```python
from build123d import *

# Parameters (mm, degrees)
F0_R     = 14
F0_R_2   = 11
F1_DEPTH = 25
F0_R_3   = 33
F2_DEPTH = 5
F3_R     = 3
F4_DEPTH = 25
F6_R     = 1
F7_DEPTH = 2


with BuildPart() as f1:
    # F0 (on Top) → F1 (new body)
    with BuildSketch(Plane.XY):
        Circle(F0_R)
        Circle(F0_R_2, mode=Mode.SUBTRACT)
    extrude(amount=F1_DEPTH)

    # F0 (on Top) → F2 (join)
    with BuildSketch(Plane.XY):
        Circle(F0_R_3)
        Circle(F0_R, mode=Mode.SUBTRACT)
    extrude(amount=F2_DEPTH)

    # F3 (on Front) → F4 (cut)
    with BuildSketch(Plane.XZ):
        with Locations((0, 25)):
            Circle(F3_R)
    extrude(amount=-F4_DEPTH, mode=Mode.SUBTRACT)

    # F6 (on offset) → F7 (join)
    with BuildSketch(Plane.XY.offset(25)):
        with Locations((-8.8388347648, 8.8388347648)):
            Circle(F6_R)
        with Locations((8.8388347648, 8.8388347648)):
            Circle(F6_R)
        with Locations((12.5, 0)):
            Circle(F6_R)
        with Locations((8.8388347648, -8.8388347648)):
            Circle(F6_R)
        with Locations((0, -12.5)):
            Circle(F6_R)
        with Locations((-8.8388347648, -8.8388347648)):
            Circle(F6_R)
        with Locations((-12.5, 0)):
            Circle(F6_R)
    extrude(amount=F7_DEPTH)


solid = f1.part
```
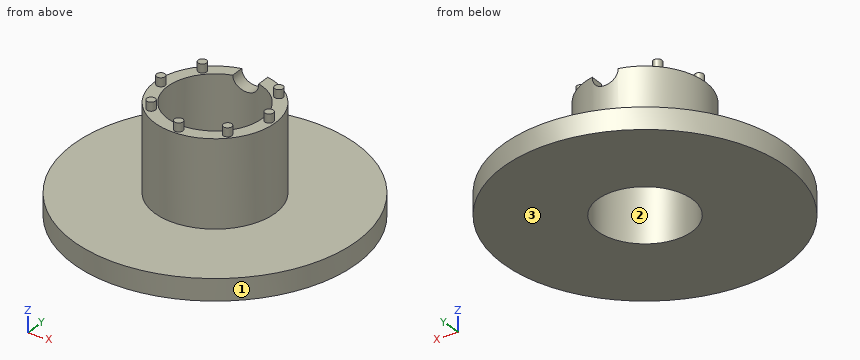
Source: CAD feature listing. Evaluate the final solid. Frame: model axes, mm. Face numbers are marked on the shaded views. Round coordinates to 2 decimals unless told otherwise and drop trailing zeros. Loops run counter-clockwise (first coordinate to the right, second up) from the corner with the lowest first, then second, coordinate; pieces in that order, holes last. Notation, with made-up numbers: M 79,53.5 L 117,53.5 A16 ccw 117,84.5 Z; hole C 84,21 d1. An arc over 180 degrees is marked long. Use a Markdown table: item, result. Add a question column.
1. Cut plane C-C, the plane z = 15. Output: boundary loops of the cut face in (x, y), and give its area (3 significant figures).
2. Pull-direction query (X, two-part tool) for the marked faces 1, 2 and 3; classes: +X half, -X half, draft (parallel to the pull), parting line (faces both ways), or undercut.
3. Cut plane B-B, the plane y = 0. Output: boundary loops of the cut face in (x, z).
4. Ray query, line 1 along Y through (x, z) = (0, 7.25); line 2 along X through (y, z) = (9, 3.75). Return the intervals inside material, ascending. Write a range as [from, to].
5. Cut plane A-A, the plane x = 0. Output: boundary loops of the cut face in (y, z).
6. Contact query for flat-ended pins moving along their axis: pin 1 (8 mm diameter, centred on x = -2.5, y = 12, fed in from +Z); pin 2 (12 mm diameter, centred on x = 8.5, z = 8.5, fed in from +Y); pin 3 (4 mm diameter, centred on x = -14.5, y = 10, fed in from -Z); pin 4 (1.5 mm diameter, centred on x = -4, z = 15.5, fed in from +Y). Output: stop coordinate, or through.
7. Cut plane D-D, the plane y = -12.5. Output: boundary loops of the cut face in (x, z).
Solution:
| question | item | result |
|---|---|---|
| 1 | outline | C 0,0 d28; hole C 0,0 d22 |
| 1 | area | 236 mm2 |
| 2 | face 1 | parting line |
| 2 | face 2 | undercut |
| 2 | face 3 | draft |
| 3 | outline | M -33,0 L -11,0 L -11,25 L -11.5,25 L -11.5,27 L -13.5,27 L -13.5,25 L -14,25 L -14,5 L -33,5 Z; M 11,0 L 33,0 L 33,5 L 14,5 L 14,25 L 13.5,25 L 13.5,27 L 11.5,27 L 11.5,25 L 11,25 Z |
| 4 | line 1 | y = [-14, -11], [11, 14] |
| 4 | line 2 | x = [-31.75, -6.32], [6.32, 31.75] |
| 5 | outline | M -33,0 L -11,0 L -11,25 L -11.5,25 L -11.5,27 L -13.5,27 L -13.5,25 L -14,25 L -14,5 L -33,5 Z; M 11,0 L 33,0 L 33,5 L 14,5 L 14,22 L 11,22 Z |
| 6 | pin 1 | stops at z = 25 |
| 6 | pin 2 | stops at y = 32.8 |
| 6 | pin 3 | stops at z = 0 |
| 6 | pin 4 | stops at y = 13.62 |
| 7 | outline | M -30.54,0 L 30.54,0 L 30.54,5 L 6.3,5 L 6.3,25 L 1,25 L 1,27 L -1,27 L -1,25 L -6.3,25 L -6.3,5 L -30.54,5 Z |
